Source: three-view drawing plus pictorial views. Frame: mm from the lowest corner of the part. A direction names the side the tool comes from. Coordinates: 2 decimals unless noted, no trailing zeros. Loops run counter-clockwise (first coordinate to the right, second up) from the corner with the lowest first, then second, coordinate; pieces in that order, holes last. Notation, with made-up numbers: (-16, -9.5) -> (7, -9.5) arc R21 cw to (7, 26.5) -> close; hole circle Ø4 at (-6.5, -36). An arc over 180 degrees is marked (long way). Answer as a JSON object with one key per item and string values. Group by question number.
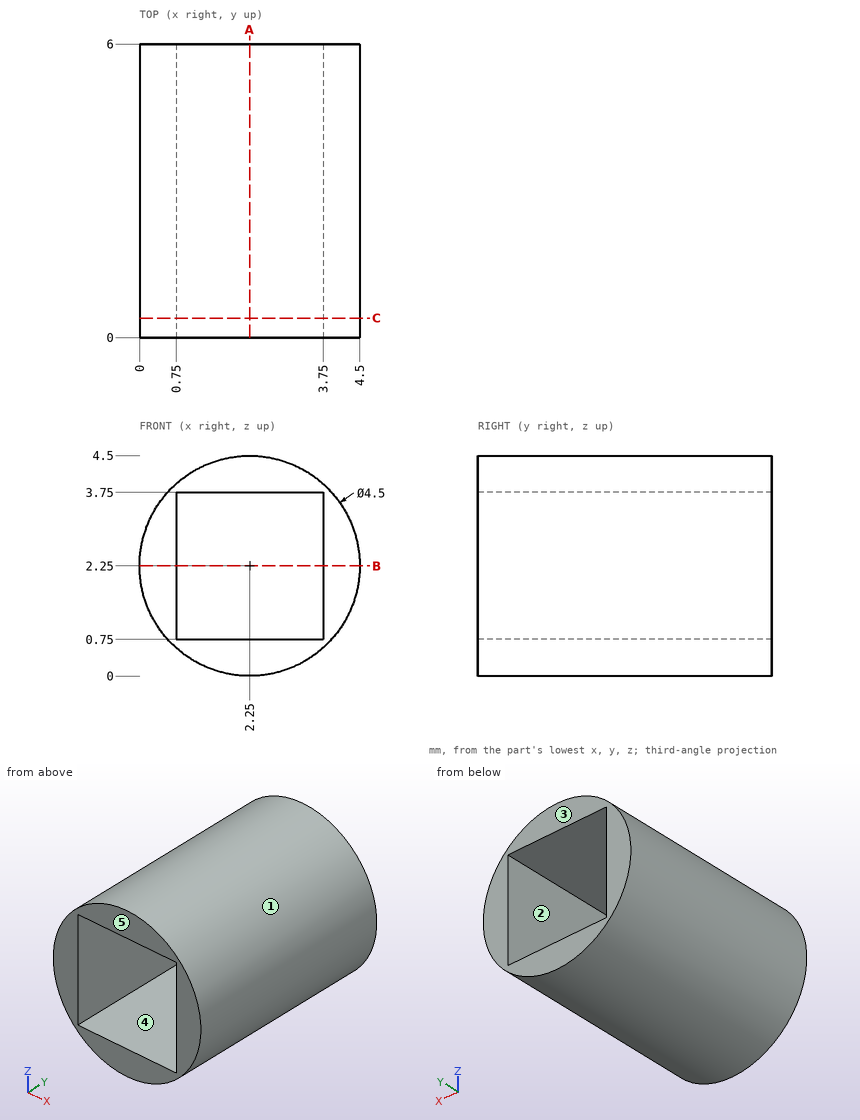
1. Reachability of the marked faces 4 and 5 from +Z, -Z, +X, -X, +Y, -Y: full face, straight path, thin tool, end or side. Return the list, or none.
2. Section query A-A on x = 2.25. Return loops of the section in (y, z).
3. Section query C-C on y = 0.4. Return loops of the section in (x, z), then the cut area to 3 significant figures.
4. Mould query, pull axis Z, two halves, no side actions, for the marked faces 1, 2 and 3. Classes: pulls with the +Z half, pulls with the -Z half, needs draft (parallel to the pull), parting line crosses it, or undercut.
5. Section query B-B on z = 2.25. Return loops of the section in (x, y).
6. Ray query, L1, parallel to X at y = 0.5, z = 2.25; L2, parallel to Z at x = 2.5, y = 0.8; L3, parallel to Z at x = 3, y = 5.55. Return the intervals inside material, ascending.
Solved:
{
 "1": {"face 4": "+Y, -Y", "face 5": "+Z, -Z, +X, -X, -Y"},
 "2": {"outline": "(0, 0) -> (6, 0) -> (6, 0.75) -> (0, 0.75) -> close; (0, 3.75) -> (6, 3.75) -> (6, 4.5) -> (0, 4.5) -> close"},
 "3": {"outline": "circle Ø4.5 at (2.25, 2.25); hole (0.75, 0.75) -> (3.75, 0.75) -> (3.75, 3.75) -> (0.75, 3.75) -> close", "area": "6.90 mm^2"},
 "4": {"face 1": "parting line crosses it", "face 2": "undercut", "face 3": "needs draft"},
 "5": {"outline": "(0, 0) -> (0.75, 0) -> (0.75, 6) -> (0, 6) -> close; (3.75, 0) -> (4.5, 0) -> (4.5, 6) -> (3.75, 6) -> close"},
 "6": {"L1": "0 to 0.75, 3.75 to 4.5", "L2": "0.01 to 0.75, 3.75 to 4.49", "L3": "0.13 to 0.75, 3.75 to 4.37"}
}
